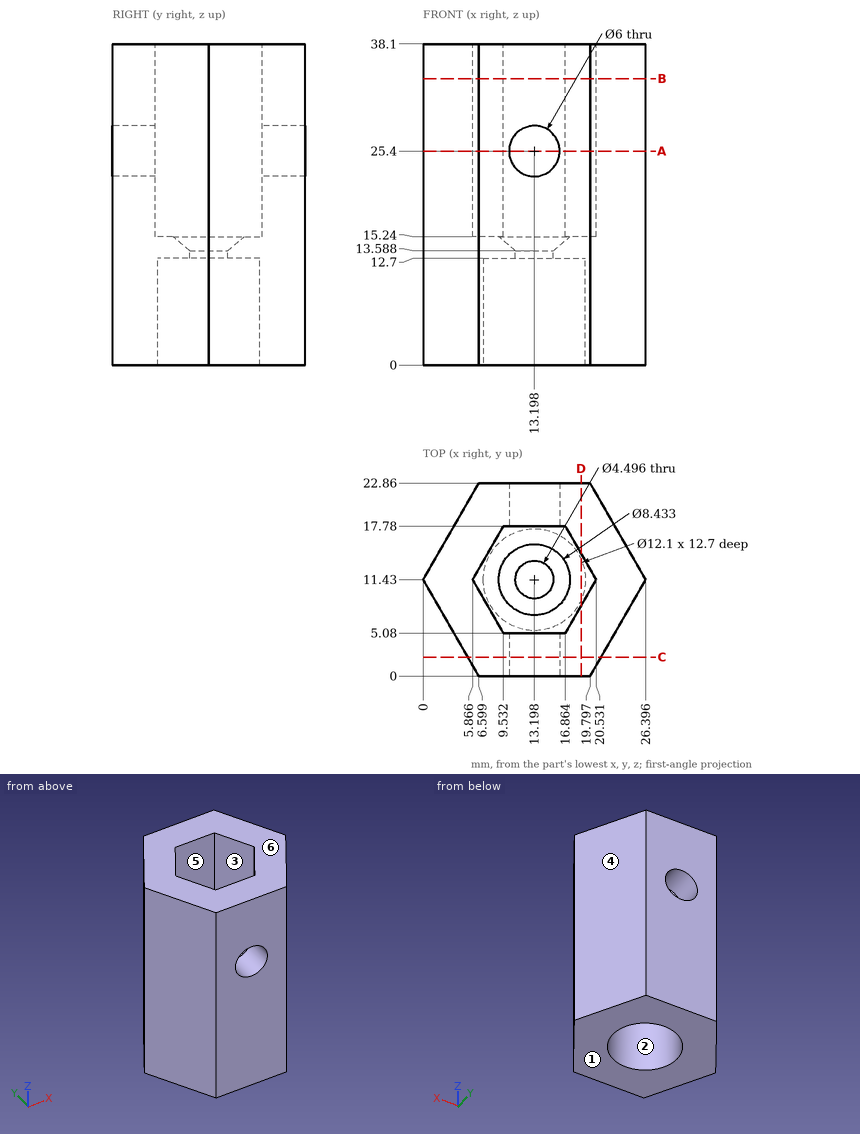
The drawing under review shows one solid part. Ordinate dimensions are in mm from its lowest x, y, z. A direction names the side the tool comes from. Round coordinates to 2 decimals unless told otherwise and drop trailing zeros. Order: outer loops, then holes, each group sorted by start corner. A loop starts at its lowest first (then second) coordinate and runs counter-clockwise, first axis right, second up. Notation, with made-up numbers: (-3.75, -22) -> (17.25, -22) arc R13 cw to (17.25, -1) -> close; hole circle Ø7 at (74.5, 33). An arc over 180 degrees is marked (long way). Use a Markdown table: item, result.
Item 1: Take a section at D-D (x = 18.75). State the section outline as (y, z) points (1 decimal), plus the area to 3 significant figures.
Resolved:
| item | result |
|---|---|
| outline | (0, 0) -> (9, 0) -> (9, 12.7) -> (13.8, 12.7) -> (13.8, 0) -> (22.9, 0) -> (22.9, 38.1) -> (14.5, 38.1) -> (14.5, 15.2) -> (8.3, 15.2) -> (8.3, 38.1) -> (0, 38.1) -> close |
| area | 669 mm² |
Item 2: Draft analysis for pull direction Y (two halves, no side actions). For the marked faces 4, 5 and 6, state which applies: +Y half, -Y half, draft (parallel to the pull), parting line (faces both ways), or undercut.
Resolved:
| item | result |
|---|---|
| face 4 | +Y half |
| face 5 | undercut |
| face 6 | draft |
Item 3: Take a section at C-C (y = 2.25). State the section outline as (x, z) points.
Resolved:
| item | result |
|---|---|
| outline | (5.3, 0) -> (21.1, 0) -> (21.1, 38.1) -> (5.3, 38.1) -> close; hole circle Ø6 at (13.2, 25.4) |
Item 4: Take a section at B-B (z = 34). State the section outline as (x, y) points (1 decimal).
Resolved:
| item | result |
|---|---|
| outline | (0, 11.4) -> (6.6, 0) -> (19.8, 0) -> (26.4, 11.4) -> (19.8, 22.9) -> (6.6, 22.9) -> close; hole (5.9, 11.4) -> (9.5, 5.1) -> (16.9, 5.1) -> (20.5, 11.4) -> (16.9, 17.8) -> (9.5, 17.8) -> close |
Item 5: For pin 1 (6 mm diameter, centred on x = 11.5, y = 11, fed in from -Z); pin 2 (12 mm diameter, centred on y = 2.5, z = 21.5, fed in from -X); pin 3 (3.5 mm diameter, centred on x = 13.2, z = 25.4, fed in from +Y); pin 4 (8 mm diameter, centred on y = 16.5, z = 21, fed in from +X), all flat-tipped, find the tip position at first contact; note any pin that passes through.
Resolved:
| item | result |
|---|---|
| pin 1 | stops at z = 12.7 |
| pin 2 | stops at x = 1.69 |
| pin 3 | passes through |
| pin 4 | stops at x = 25.78 |
Item 6: Take a section at A-A (z = 25.4). State the section outline as (x, y) points (1 decimal).
Resolved:
| item | result |
|---|---|
| outline | (0, 11.4) -> (6.6, 0) -> (10.2, 0) -> (10.2, 5.1) -> (9.5, 5.1) -> (5.9, 11.4) -> (9.5, 17.8) -> (10.2, 17.8) -> (10.2, 22.9) -> (6.6, 22.9) -> close; (16.2, 0) -> (19.8, 0) -> (26.4, 11.4) -> (19.8, 22.9) -> (16.2, 22.9) -> (16.2, 17.8) -> (16.9, 17.8) -> (20.5, 11.4) -> (16.9, 5.1) -> (16.2, 5.1) -> close |
Item 7: Machinability: for the marked faces 1, 2 and 3, which of the approach directions +Z, -Z, +X, -X, +Y, -Y give a long, thin tool a straight path to every point of the face, cutting with its end or side? Answer none if there is none.
Resolved:
| item | result |
|---|---|
| face 1 | -Z, +X, -X, +Y, -Y |
| face 2 | -Z |
| face 3 | +Z |
Item 8: For line 1 along Y through (x, z) = (12.5, 34.5); line 2 along Y through (x, z) = (10.25, 8.5); line 3 along Z through (x, y) = (13.5, 20.5) (1 decimal), list the stretches that pass through material, from the lowest coordinate up. Write a range as [from, to].
Resolved:
| item | result |
|---|---|
| line 1 | y = [0, 5.08], [17.78, 22.86] |
| line 2 | y = [0, 6.15], [16.71, 22.86] |
| line 3 | z = [0, 22.4], [28.4, 38.1] |
